Source: CAD feature listing. Evaluate the final solid. Frame: model axes, mm. Give positions to 0.01 mm unless a question says otherwise; leave off trailing zeros. Loops run counter-clockwise (first coordinate to the right, second up) from the corner with the lowest first, then second, coordinate; pieces in that order, holes last. Notation, with made-up numbers: (-16, -3.5) -> (32, -3.5) arc R20 cw to (32, 0.5) -> close; hole circle Ø8 at (-15.75, 30). An arc over 180 degrees is marked (long way). Answer as a JSON object with one key per item and string values. Group by question number.
from build123d import *

# Parameters (mm, degrees)
F0_W      = 44.656470418
F0_H      = 33.8078811765
F1_DEPTH  = 16
F2_DEPTH  = 796
F3_DEPTH  = 196
F4_W      = 68.9578056335
F4_H      = 493.6993122101
F5_DEPTH  = 7
F6_DEPTH  = 9.7
F7_DEPTH  = 99.33
F8_DEPTH  = 99.33
F9_DEPTH  = 17.34
F10_DEPTH = 102.97
F11_W     = 35.2807044983
F11_H     = 492.0964837074
F12_DEPTH = 7
F13_DEPTH = 37.27
F14_DEPTH = 6.58
F15_DEPTH = 106.63
F16_DEPTH = 5.87
F17_DEPTH = 200
F18_DEPTH = 200
F19_DEPTH = 200
F20_DEPTH = 600
F21_DEPTH = 600
F22_DEPTH = 600
F23_DEPTH = 200
F24_DEPTH = 200
F25_DEPTH = 200
F26_R     = 3


with BuildPart() as f1:
    # F0 (on Front) → F1 (new body)
    with BuildSketch(Plane.XZ):
        with Locations((22.328235209, 16.9039405882)):
            Rectangle(F0_W, F0_H)
    extrude(amount=F1_DEPTH)

    # F2 (add): a face of the model
    f2_faces = [f1.faces().sort_by_distance(p)[0] for p in [
        (22.328235209, -8, 0),
    ]]
    extrude(f2_faces, amount=-F2_DEPTH)

    # F3 (add): a face of the model
    f3_faces = [f1.faces().sort_by_distance(p)[0] for p in [
        (0, -8, 398),
    ]]
    extrude(f3_faces, amount=-F3_DEPTH)

    # F4 (on face) → F5 (cut)
    with BuildSketch(Plane.XZ.offset(16)):
        with Locations((94.1769480705, 399.8196721077)):
            Rectangle(F4_W, F4_H)
    extrude(amount=-F5_DEPTH, mode=Mode.SUBTRACT)

    # F6 (cut): a face of the model
    f6_faces = [f1.faces().sort_by_distance(p)[0] for p in [
        (59.6980452538, -12.5, 399.8196721077),
    ]]
    extrude(f6_faces, amount=-F6_DEPTH, mode=Mode.SUBTRACT)

    # F7 (add): a face of the model
    f7_faces = [f1.faces().sort_by_distance(p)[0] for p in [
        (89.3269480705, -12.5, 646.6693282127),
    ]]
    extrude(f7_faces, amount=-F7_DEPTH)

    # F8 (cut): a face of the model
    f8_faces = [f1.faces().sort_by_distance(p)[0] for p in [
        (89.3269480705, -12.5, 646.6693282127),
    ]]
    extrude(f8_faces, amount=-F8_DEPTH, mode=Mode.SUBTRACT)

    # F9 (cut): a face of the model
    f9_faces = [f1.faces().sort_by_distance(p)[0] for p in [
        (128.6558508873, -12.5, 449.4846721077),
    ]]
    extrude(f9_faces, amount=-F9_DEPTH, mode=Mode.SUBTRACT)

    # F10 (cut): a face of the model
    f10_faces = [f1.faces().sort_by_distance(p)[0] for p in [
        (97.9969480705, -12.5, 152.9700160027),
    ]]
    extrude(f10_faces, amount=-F10_DEPTH, mode=Mode.SUBTRACT)

    # F11 (on face) → F12 (join)
    with BuildSketch(Plane.XZ.offset(9)):
        with Locations((91.7714834213, 432.6795041561)):
            Rectangle(F11_W, F11_H)
    extrude(amount=F12_DEPTH)

    # F13 (add): a face of the model
    f13_faces = [f1.faces().sort_by_distance(p)[0] for p in [
        (91.7714834213, -12.5, 678.7277460098),
    ]]
    extrude(f13_faces, amount=F13_DEPTH)

    # F14 (add): a face of the model
    f14_faces = [f1.faces().sort_by_distance(p)[0] for p in [
        (109.4118356705, -12.5, 451.3145041561),
    ]]
    extrude(f14_faces, amount=F14_DEPTH)

    # F15 (add): a face of the model
    f15_faces = [f1.faces().sort_by_distance(p)[0] for p in [
        (95.0614834213, -12.5, 186.6312623024),
    ]]
    extrude(f15_faces, amount=F15_DEPTH)

    # F16 (cut): a face of the model
    f16_faces = [f1.faces().sort_by_distance(p)[0] for p in [
        (74.1311311722, -12.5, 397.9995041561),
    ]]
    extrude(f16_faces, amount=-F16_DEPTH, mode=Mode.SUBTRACT)

    # F17 (add): a face of the model
    f17_faces = [f1.faces().sort_by_distance(p)[0] for p in [
        (196, -8, 398),
    ]]
    extrude(f17_faces, amount=F17_DEPTH)

    # F18 (cut): a face of the model
    f18_faces = [f1.faces().sort_by_distance(p)[0] for p in [
        (145.9958508873, -12.5, 397.9996721077),
    ]]
    extrude(f18_faces, amount=-F18_DEPTH, mode=Mode.SUBTRACT)

    # F19 (add): a face of the model
    f19_faces = [f1.faces().sort_by_distance(p)[0] for p in [
        (115.9918356705, -12.5, 397.9995041561),
    ]]
    extrude(f19_faces, amount=F19_DEPTH)

    # F20 (cut): a face of the model
    f20_faces = [f1.faces().sort_by_distance(p)[0] for p in [
        (197.9964834213, -12.5, 80.0012623024),
    ]]
    extrude(f20_faces, amount=-F20_DEPTH, mode=Mode.SUBTRACT)

    # F21 (add): a face of the model
    f21_faces = [f1.faces().sort_by_distance(p)[0] for p in [
        (197.9969480705, -12.5, 50.0000160027),
    ]]
    extrude(f21_faces, amount=F21_DEPTH)

    # F22 (cut): a face of the model
    f22_faces = [f1.faces().sort_by_distance(p)[0] for p in [
        (198, -8, 0),
    ]]
    extrude(f22_faces, amount=-F22_DEPTH, mode=Mode.SUBTRACT)

    # F23 (add): a face of the model
    f23_faces = [f1.faces().sort_by_distance(p)[0] for p in [
        (198, -8, 600),
    ]]
    extrude(f23_faces, amount=F23_DEPTH)

    # F24 (cut): a face of the model
    f24_faces = [f1.faces().sort_by_distance(p)[0] for p in [
        (197.9969480705, -12.5, 650.0000160027),
    ]]
    extrude(f24_faces, amount=-F24_DEPTH, mode=Mode.SUBTRACT)

    # F25 (add): a face of the model
    f25_faces = [f1.faces().sort_by_distance(p)[0] for p in [
        (197.9964834213, -12.5, 680.0012623024),
    ]]
    extrude(f25_faces, amount=F25_DEPTH)

    # F26
    f26_edges = [f1.edges().sort_by_distance(p)[0] for p in [
        (197.996483, -16, 480.001262),
        (80.001131, -16, 597.999504),
        (197.996483, -16, 715.997746),
        (315.991836, -16, 597.999504),
        (0, -16, 598),
        (198, -16, 400),
        (396, -16, 598),
        (198, -16, 796),
        (49.998045, -16, 597.999672),
        (197.996948, -16, 745.999328),
        (345.995851, -16, 597.999672),
        (197.996948, -16, 450.000016),
    ]]
    fillet(f26_edges, radius=F26_R)


solid = f1.part
(1) Section query A-A on z = 469. Return the cut outline in (x, y), plus the area to 3 significant figures.
(2) Section query B-B on x = 104.5. Return the cut outline in (y, z).
(3) Section query C-C on z = 565. Return the cut outline in (x, y).
(4) Mould query, pull axis X, two halves, no side actions, for faces 1 (the face through (396, -6, 601)), 2 (the face through (327, -9, 596)), 3 (the face through (0, -6, 601)), 4 (the face through (195, -6, 400)). Classes: pulls with the +X half, pulls with the -X half, needs draft (parallel to the pull), parting line crosses it, or undercut.
(5) Material intervals for line 1 (Z direction, x = 163, y = -10.5); line 2 (Z direction, x = 52, y = -11.25); line 3 (Y direction, x = 69.5, z = 615.5), sorted ascending. Write a range as from..to.
Result:
{
 "1": {"outline": "(0, -13) arc R3 ccw to (3, -16) -> (47, -16) arc R3 ccw to (50, -13) -> (50, -9) -> (346, -9) -> (346, -13) arc R3 ccw to (349, -16) -> (393, -16) arc R3 ccw to (396, -13) -> (396, 0) -> (0, 0) -> close", "area": "4,260 mm²"},
 "2": {"outline": "(-16, 403) arc R3 ccw to (-13, 400) -> (0, 400) -> (0, 796) -> (-13, 796) arc R3 ccw to (-16, 793) -> (-16, 749) arc R3 ccw to (-13, 746) -> (-9, 746) -> (-9, 716) -> (-13, 716) arc R3 ccw to (-16, 713) -> (-16, 483) arc R3 ccw to (-13, 480) -> (-9, 480) -> (-9, 450) -> (-13, 450) arc R3 ccw to (-16, 447) -> close"},
 "3": {"outline": "(0, -13) arc R3 ccw to (3, -16) -> (47, -16) arc R3 ccw to (50, -13) -> (50, -9) -> (80, -9) -> (80, -13) arc R3 ccw to (83, -16) -> (312.99, -16) arc R3 ccw to (315.99, -13) -> (315.99, -9) -> (346, -9) -> (346, -13) arc R3 ccw to (349, -16) -> (393, -16) arc R3 ccw to (396, -13) -> (396, 0) -> (0, 0) -> close"},
 "4": {"face 1": "pulls with the +X half", "face 2": "undercut", "face 3": "pulls with the -X half", "face 4": "needs draft"},
 "5": {"line 1": "400..450, 480..716, 746..796", "line 2": "400..450, 746..796", "line 3": "-9..0"}
}
